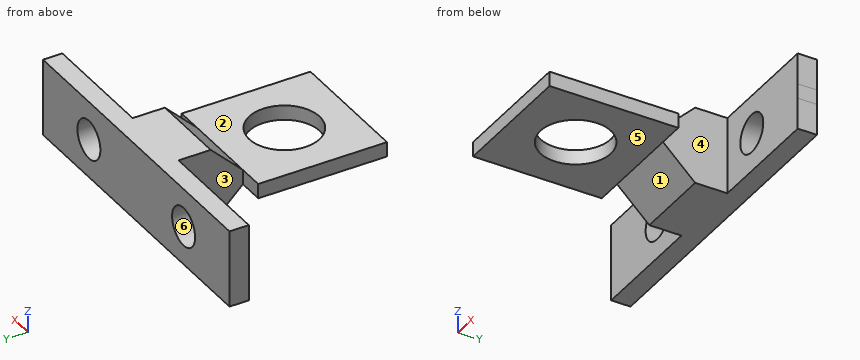
from build123d import *

# Parameters (mm, degrees)
SALIENTE_EXTRUIR1_DEPTH = 2.286
CROQUIS3_W              = 12
CROQUIS3_H              = 3
SALIENTE_EXTRUIR2_DEPTH = 48.748737
SALIENTE_EXTRUIR3_DEPTH = 12
CROQUIS5_R              = 5.46
CORTAR_EXTRUIR1_DEPTH   = 8.143
CROQUIS6_R              = 3
CORTAR_EXTRUIR2_DEPTH   = 3


with BuildPart() as part:
    # Croquis1 → Saliente-Extruir1 (new body)
    with BuildSketch(Plane.XY):
        Polygon((-14.666527812, 16.476832902), (-63.415265152, 16.476832902), (-63.415265152, 13.476832902), (-45.040896482, 13.476832902), (-45.040896482, 8.476832902), (-45.040896482, 3.476832902), (-49.040896482, 3.476832902), (-49.040896482, -16.523167098), (-29.040896482, -16.523167098), (-29.040896482, 3.476832902), (-33.040896482, 3.476832902), (-33.040896482, 8.476832902), (-33.040896482, 13.476832902), (-14.666527812, 13.476832902), align=None)
    extrude(amount=SALIENTE_EXTRUIR1_DEPTH)

    # Croquis3 → Saliente-Extruir2 (add)
    with BuildSketch(Plane.ZY.offset(63.415265152)):
        with Locations((1.143, 14.976832902)):
            Rectangle(CROQUIS3_W, CROQUIS3_H)
    extrude(amount=-SALIENTE_EXTRUIR2_DEPTH)

    # Croquis4 → Saliente-Extruir3 (add)
    with BuildSketch(Plane(origin=(-33.040896482, 0, 0), x_dir=(0, 0, -1), z_dir=(1, 0, 0))):
        Polygon((4.857, 8.476832902), (0, 3.476832902), (-2.286, 3.476832902), (-7.143, 8.476832902), (-7.143, 13.476832902), (4.857, 13.476832902), align=None)
    extrude(amount=-SALIENTE_EXTRUIR3_DEPTH)

    # Croquis5 → Cortar-Extruir1 (cut, through all)
    with BuildSketch(Plane.XY.offset(2.286)):
        with Locations((-39.040896482, -6.523167098)):
            Circle(CROQUIS5_R)
    extrude(amount=-CORTAR_EXTRUIR1_DEPTH, mode=Mode.SUBTRACT)

    # Croquis6 → Cortar-Extruir2 (cut)
    with BuildSketch(Plane(origin=(0, 16.476832902, 0), x_dir=(1, 0, 0), z_dir=(0, 1, 0))):
        with Locations((-26.666527812, -1.143)):
            Circle(CROQUIS6_R)
        with Locations((-51.415265152, -1.143)):
            Circle(CROQUIS6_R)
    extrude(amount=-CORTAR_EXTRUIR2_DEPTH, mode=Mode.SUBTRACT)


solid = part.part
Read the model definition and answer for the solid it produces. Units are mm, in the model's axes. Face numbers are marked on the shaded views. A direction names the side the tool comes from. Coordinates: 2 decimals unless noted, no trailing zeros. Order: outer loops, then holes, each group sorted by start corner. A loop starts at its lowest first (then second) coordinate and runs counter-clockwise, first axis right, second up. Notation, with made-up numbers: (-32, 75.5) - (16, 75.5) arc R19 ccw to (16, 100.5) - close; hole circle Ø9 at (24, 82). An arc over 180 degrees is marked (long way). Use one line per item in the form item = value.
(1) Section C-C, the plane z = 3.25 is taken. Give the vertices of the cut face in (x, y).
Computed values:
outline = (-63.42, 13.48) - (-53.55, 13.48) - (-53.55, 16.48) - (-63.42, 16.48) - close; (-49.28, 13.48) - (-45.04, 13.48) - (-45.04, 4.47) - (-33.04, 4.47) - (-33.04, 13.48) - (-28.8, 13.48) - (-28.8, 16.48) - (-49.28, 16.48) - close; (-24.53, 13.48) - (-14.67, 13.48) - (-14.67, 16.48) - (-24.53, 16.48) - close
(2) Section D-D, the plane y = -12.5 is taken. Give the vertices of the cut face in (x, z), then the cut area to 3 significant figures.
Computed values:
outline = (-49.04, 0) - (-29.04, 0) - (-29.04, 2.29) - (-49.04, 2.29) - close
area = 45.7 mm²
(3) Given pin 1 Ø1.8 at (y, z) = (-6.5, 0.5) entering from +X; pin 2 Ø10 at (x, y) = (-37.5, -2) entering from +Z; pin 3 Ø2 at (x, z) = (-32, -2) entering from -Y, each flat-ended and moving along its own axis, determine where each tip first touches the part or whether it passes through.
Computed values:
pin_1 = -29.04
pin_2 = 2.29
pin_3 = 13.48
(4) Section A-A, the plane x = -31.5 is taken. Give the vertices of the cut face in (y, z), then the cut area to 3 significant figures.
Computed values:
outline = (-16.52, 0) - (3.48, 0) - (3.48, 2.29) - (-16.52, 2.29) - close; (13.48, -4.86) - (16.48, -4.86) - (16.48, 7.14) - (13.48, 7.14) - close
area = 81.7 mm²
(5) Section B-B, the plane z = 0.5 is taken. Give the vertices of the cut face in (x, y), then the cut area to 3 significant figures.
Computed values:
outline = (-63.42, 13.48) - (-54.35, 13.48) - (-54.35, 16.48) - (-63.42, 16.48) - close; (-49.04, -16.52) - (-29.04, -16.52) - (-29.04, 3.48) - (-33.04, 3.48) - (-33.04, 13.48) - (-29.6, 13.48) - (-29.6, 16.48) - (-48.48, 16.48) - (-48.48, 13.48) - (-45.04, 13.48) - (-45.04, 3.48) - (-49.04, 3.48) - close; (-23.74, 13.48) - (-14.67, 13.48) - (-14.67, 16.48) - (-23.74, 16.48) - close; hole circle Ø10.92 at (-39.04, -6.52)
area = 537 mm²
(6) Which of the six approach directions +Z, -Z, +X, -X, +Y, -Y give full straight-line access (tool end or side, diameter ignored) to the marked faces 1, 2 and 3?
Computed values:
face_1 = -Z, +X, -X, -Y
face_2 = +Z, +X, -X, -Y
face_3 = +Z, -Z, -X
(7) Straight lines are drawn through the part: L1, parallel to X at y = 12.5, z = 4; L2, parallel to Y at x = -26, z = -3; L3, parallel to Z at x = -29.5, y = -2.5. For each, find the intervals that lie inside material, in ascending order.
Computed values:
L1 = -45.04 to -33.04
L2 = 13.48 to 16.48
L3 = 0 to 2.29
(8) For a pull along X with two mould halves and no side action, classify the marked faces 4, 5 and 6 as pulls with the +X half, pulls with the -X half, needs draft (parallel to the pull), parting line crosses it, or undercut.
Computed values:
face_4 = pulls with the +X half
face_5 = needs draft
face_6 = undercut
